from build123d import *

# Parameters (mm, degrees)
SKETCH1_W           = 25.4
SKETCH1_H           = 50.8
SKETCH1_W_2         = 21.4
SKETCH1_H_2         = 46.8
BOSS_EXTRUDE1_DEPTH = 250
SKETCH2_W           = 80
SKETCH2_H           = 46
CUT_EXTRUDE1_DEPTH  = 20


with BuildPart() as part:
    # Sketch1 → Boss-Extrude1 (new body)
    with BuildSketch(Plane.XY):
        Rectangle(SKETCH1_W, SKETCH1_H)
        Rectangle(SKETCH1_W_2, SKETCH1_H_2, mode=Mode.SUBTRACT)
    extrude(amount=BOSS_EXTRUDE1_DEPTH)

    # Sketch2 → Cut-Extrude1 (cut)
    with BuildSketch(Plane.ZY.offset(12.7)):
        with Locations((40, 0)):
            Rectangle(SKETCH2_W, SKETCH2_H)
        with Locations((210, 0)):
            Rectangle(SKETCH2_W, SKETCH2_H)
    extrude(amount=-CUT_EXTRUDE1_DEPTH, mode=Mode.SUBTRACT)


solid = part.part
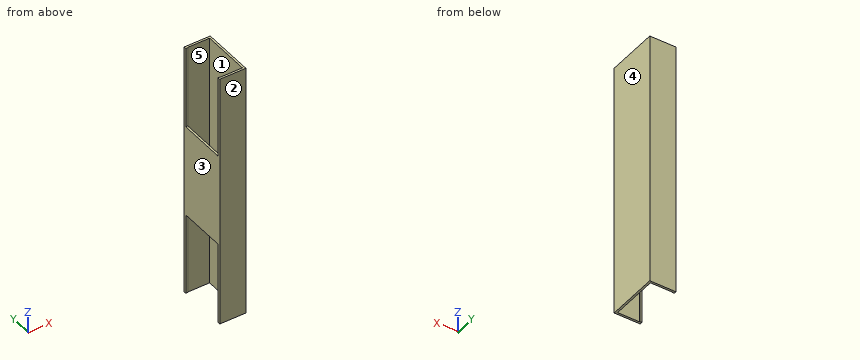
Input: part model. Units: mm. Frame: model coordinates. Face numbers are marked on the shaded views. A direction names the side the tool comes from. Coordinates: 2 decimals unless noted, no trailing zeros. Loops run counter-clockwise (first coordinate to the right, second up) from the corner with the lowest first, then second, coordinate; pieces in that order, holes last.
(1) Material intervals for probe 1 along Y at (x, z) = (-2, 106.5); probe 2 along Y at (x, z) = (-10.75, 16.5); probe 3 along X at (y, z) = (5.5, 102.5), sorted ascending.
(2) First-contact query: pin 1 Ø8 at (x, y) = (-9, -12.5) entering from +Z; pin 2 Ø10 at (y, z) = (15, 43.5) entering from -X; pin 3 Ø2 at (x, y) = (-11, 0.5) entering from -Z; pin 4 Ø8 at (x, y) = (-3, -15) entering from +Z. Flat tips, straight axial feed; report the tip coordinate or a pass-through.
(3) Section C-C on y = 14. Return the cut outline in (x, z).
(4) Section D-D on z = 59.5. Return the cut outline in (x, y).
(5) Set-up query: the marked faces 4 and 5. Return all of +Z, -Z, +X, -X, +Y, -Y with unobstructed straight access to the full face (end or side cutting, diameter ignored); none if empty.
(6) Section A-A on x = 5.25. Return the cut outline in (y, z).
(7) Pull-direction query (X, two-part tool) for the marked faces 1, 2 and 3; classes: released by +X, released by -X, zero draft, split by the parting line, or undercut.
(8) Section B-B on z = 152.5. Return the cut outline in (x, y).
Data:
1. probe 1: y = -25.4 to -23.4, 23.4 to 25.4
1. probe 2: y = -25.4 to -23, 23 to 25.4
1. probe 3: x = -12.7 to -10.7, 10.7 to 12.7
2. pin 1: stops at z = 170
2. pin 2: stops at x = 10.7
2. pin 3: stops at z = 80
2. pin 4: passes through
3. outline: (-12.7, 80) - (-10.7, 80) - (-10.7, 170) - (-12.7, 170) - close; (10.7, 0) - (12.7, 0) - (12.7, 250) - (10.7, 250) - close
4. outline: (-12.7, -25.4) - (12.7, -25.4) - (12.7, 25.4) - (-12.7, 25.4) - (-12.7, 23) - (-10.7, 23) - (-10.7, 23.4) - (10.7, 23.4) - (10.7, -23.4) - (-10.7, -23.4) - (-10.7, -23) - (-12.7, -23) - close
5. face 4: +Z, -Z, +X, +Y, -Y
5. face 5: +Z, -Z
6. outline: (-25.4, 0) - (-23.4, 0) - (-23.4, 250) - (-25.4, 250) - close; (23.4, 0) - (25.4, 0) - (25.4, 250) - (23.4, 250) - close
7. face 1: undercut
7. face 2: zero draft
7. face 3: released by -X
8. outline: (-12.7, -25.4) - (12.7, -25.4) - (12.7, 25.4) - (-12.7, 25.4) - close; hole (-10.7, -23.4) - (10.7, -23.4) - (10.7, 23.4) - (-10.7, 23.4) - close
